from build123d import *

# Parameters (mm, degrees)
PAD_DEPTH         = 22
SKETCH001_R       = 3.1
POCKET_DEPTH      = 5.001
POCKET_DEPTH_BACK = -27.001
SKETCH002_R       = 3.1
POCKET001_DEPTH   = 5
SKETCH003_R       = 1.6
POCKET002_DEPTH   = 44.001
FILLET_R          = 2
SKETCH004_R       = 1.95
POCKET003_DEPTH   = 5


with BuildPart() as part:
    # Sketch → Pad (new body, symmetric)
    with BuildSketch(Plane.XZ):
        Polygon((0, 27), (0, 0), (27, 0), (27, -5), (-32, -5), (-32, 7), (-5, 7), (-5, 27), align=None)
    extrude(amount=PAD_DEPTH, both=True)

    # Sketch001 → Pocket (cut, two sides)
    with BuildSketch(Plane.XY) as pocket_sk:
        with Locations((15, 12.5)):
            Circle(SKETCH001_R)
        with Locations((15, -12.5)):
            Circle(SKETCH001_R)
        with BuildLine():
            ThreePointArc((-16.803848, -3), (-26.859933, 3.518672), (-17.527864, -4))
            Line((-6, -4), (-17.527864, -4))
            Line((-6, -4), (-6, -10))
            Line((-6, -10), (-22, -10))
            ThreePointArc((-29.660444, 6.427876), (-31.063078, -4.226183), (-22, -10))
            Line((-18.392302, 19.856726), (-29.660444, 6.427876))
            ThreePointArc((-13.796055, 22), (-16.331753, 21.437843), (-18.392302, 19.856726))
            Line((-13.796055, 22), (-13.796055, 28.799225))
            Line((-13.796055, 28.799225), (-40.339119, 28.799225))
            Line((-40.339119, 28.799225), (-40.339119, -28.958258))
            Line((-40.339119, -28.958258), (-5, -28.958258))
            Line((-5, -28.958258), (-5, -3))
            Line((-16.803848, -3), (-5, -3))
        make_face()
    extrude(amount=-POCKET_DEPTH, mode=Mode.SUBTRACT)
    extrude(pocket_sk.sketch, amount=-POCKET_DEPTH_BACK, mode=Mode.SUBTRACT)

    # Sketch002 → Pocket001 (cut)
    with BuildSketch(Plane.YZ):
        with Locations((-12.5, 15)):
            Circle(SKETCH002_R)
        with Locations((12.5, 15)):
            Circle(SKETCH002_R)
    extrude(amount=-POCKET001_DEPTH, mode=Mode.SUBTRACT)

    # Sketch003 (on Face5 of Pocket001) → Pocket002 (cut, through all)
    with BuildSketch(Plane(origin=(0, 22, 0), x_dir=(1, 0, 0), z_dir=(0, 1, 0))):
        with Locations((-11, -1)):
            Circle(SKETCH003_R)
    extrude(amount=-POCKET002_DEPTH, mode=Mode.SUBTRACT)

    # Fillet
    fillet_edges = [part.edges().sort_by_distance(p)[0] for p in [
        (-6, -4, 1),
        (-6, -10, 1),
        (-5, -3, 1),
        (-5, 9.5, 7),
        (27, -22, -2.5),
        (27, 22, -2.5),
        (0, 0, 0),
        (-2.5, -22, 27),
        (-2.5, 22, 27),
    ]]
    fillet(fillet_edges, radius=FILLET_R)

    # Sketch004 (on Face2 of Fillet) → Pocket003 (cut)
    with BuildSketch(Plane(origin=(0, 22, 0), x_dir=(1, 0, 0), z_dir=(0, 1, 0))):
        with Locations((-11, -1)):
            Circle(SKETCH004_R)
    extrude(amount=-POCKET003_DEPTH, mode=Mode.SUBTRACT)


solid = part.part
Design review of the part built by this model. Coordinates are the model's own, in mm. A direction names the side the tool comes from. Give positions to 0.01 mm unless a question says otherwise; leave off trailing zeros. Loops run counter-clockwise (first coordinate to the right, second up) from the corner with the lowest first, then second, coordinate; pieces in that order, holes last. Notation, with made-up numbers: (-20, -32.75) - (22, -32.75) arc R25 cw to (22, -12.75) - close; hole circle Ø8 at (76, -1). An arc over 180 degrees is marked (long way). Use CSV: the item, a comma, the result in double quotes. Start each with the question number.
1. Machinability: for faces 1 (the flat face through (-13, -4, 1)), 2 (the cylindrical face through (-6.57, -9.4, 1.08)), 3 (the cylindrical face through (-9.14, 19.54, 0.41)), which of the approach directions +Z, -Z, +X, -X, +Y, -Y give a long, thin tool a straight path to every point of the face, cutting with its end or side? Answer none if there is none.
2. Draft analysis for pull direction Y (two halves, no side actions). For faces 4 (the flat face through (-6, -7, 1)), 5 (the cylindrical face through (-2.46, 21.4, 26.43)), 6 (the cylindrical face through (-6.6, -4.57, 1.08)), state which applies: released by +Y, released by -Y, zero draft, split by the parting line, or undercut.
3. Add section B-B (z = 15). State the section outline as (x, y) points, plus the area to 3 significant figures.
4. Add section C-C (x = 15). State the section outline as (y, z) points, plus the area to 3 significant figures.
5. Wall thickness on L1, parallel to Y at x = 15, z = -1; L2, parallel to Z at x = -11, y = 4.5; L3, parallel to Z at x = -3.05, y = -12.5: over which ranges is each line inside the solid? List them lowest first.
6. Insertion check: P1, Ø2, axis at x = -12.5, z = -1.5, coming from the -Y side; P2, Ø4, axis at y = -12.5, z = 6, coming from the -X side; P3, Ø0.6, axis at y = -7.5, z = 4, coming from the +X side. Each pin has a flat end and moves straight along its axis. Give the tip position at first contact, or say it passes through.
7. Add section A-A (y = 4.5). State the section outline as (x, z) points.
8. Add section D-D (y = 12.5). State the section outline as (x, z) points.
Results found:
1,face 1,"+Z, -Z"
1,face 2,"+Z, -Z, -Y"
1,face 3,"+Y"
2,face 4,"zero draft"
2,face 5,"released by +Y"
2,face 6,"undercut"
3,outline,"(-5, -22) - (0, -22) - (0, -15.6) - (-5, -15.6) - close; (-5, -9.4) - (0, -9.4) - (0, 9.4) - (-5, 9.4) - close; (-5, 15.6) - (0, 15.6) - (0, 22) - (-5, 22) - close"
3,area,"158 mm²"
4,outline,"(-22, -5) - (-15.6, -5) - (-15.6, 0) - (-22, 0) - close; (-9.4, -5) - (9.4, -5) - (9.4, 0) - (-9.4, 0) - close; (15.6, -5) - (22, -5) - (22, 0) - (15.6, 0) - close"
4,area,"158 mm²"
5,L1,"y = -22 to -15.6, -9.4 to 9.4, 15.6 to 22"
5,L2,"z = -5 to -0.6, 2.6 to 7"
5,L3,"z = -5 to 11.9, 18.1 to 27"
6,P1,"stops at y = -10"
6,P2,"stops at x = -5"
6,P3,"stops at x = 0"
7,outline,"(-30.93, -5) - (-25.97, -5) - (-25.97, 7) - (-30.93, 7) - close; (-18.03, -5) - (27, -5) - (27, 0) - (2, 0) arc R2 cw to (0, 2) - (0, 27) - (-5, 27) - (-5, 9) arc R2 cw to (-7, 7) - (-18.03, 7) - close; hole circle Ø3.2 at (-11, 1)"
8,outline,"(-24.57, -5) - (11.9, -5) - (11.9, 0) - (2, 0) arc R2 cw to (0, 2) - (0, 11.9) - (-5, 11.9) - (-5, 9) arc R2 cw to (-7, 7) - (-24.57, 7) - close; (-5, 18.1) - (0, 18.1) - (0, 27) - (-5, 27) - close; (18.1, -5) - (27, -5) - (27, 0) - (18.1, 0) - close; hole circle Ø3.2 at (-11, 1)"
